from build123d import *

# Parameters (mm, degrees)
SKETCH1_W                      = 40
SKETCH1_H                      = 10.5
BOSS_EXTRUDE1_DEPTH            = 2
SKETCH2_W                      = 14.65
SKETCH2_H                      = 10.5
SKETCH2_W_2                    = 5.2
BOSS_EXTRUDE2_DEPTH            = 3
SKETCH3_W                      = 25
SKETCH3_H                      = 18
BOSS_EXTRUDE3_DEPTH            = 12
CBORE_FOR_M5_SHCS1_D           = 5.5
CBORE_FOR_M5_SHCS1_DEPTH       = 12
CBORE_FOR_M5_SHCS1_CBORE_D     = 10.5
CBORE_FOR_M5_SHCS1_CBORE_DEPTH = 6
FILLET1_R                      = 3
SKETCH6_R                      = 0.95
CUT_EXTRUDE1_DEPTH             = 23


with BuildPart() as part:
    # Sketch1 → Boss-Extrude1 (new body)
    with BuildSketch(Plane.XY):
        with Locations((-20, 5.25)):
            Rectangle(SKETCH1_W, SKETCH1_H)
    extrude(amount=BOSS_EXTRUDE1_DEPTH)

    # Sketch2 → Boss-Extrude2 (add)
    with BuildSketch(Plane.XY.offset(2)):
        with Locations((-32.675, 5.25)):
            Rectangle(SKETCH2_W, SKETCH2_H)
        with Locations((-2.6, 5.25)):
            Rectangle(SKETCH2_W_2, SKETCH2_H)
    extrude(amount=BOSS_EXTRUDE2_DEPTH)

    # Sketch3 → Boss-Extrude3 (add)
    with BuildSketch(Plane(origin=(0, 0, 0), x_dir=(0, 0, -1), z_dir=(1, 0, 0))):
        with Locations((7.5, 9)):
            Rectangle(SKETCH3_W, SKETCH3_H)
    extrude(amount=BOSS_EXTRUDE3_DEPTH)

    # CBORE for M5 SHCS1
    with Locations(Plane(origin=(12, 0, 0), x_dir=(0, 0, -1), z_dir=(1, 0, 0))):
        with Locations((10, 6)):
            CounterBoreHole(CBORE_FOR_M5_SHCS1_D / 2, CBORE_FOR_M5_SHCS1_CBORE_D / 2, CBORE_FOR_M5_SHCS1_CBORE_DEPTH, depth=CBORE_FOR_M5_SHCS1_DEPTH)

    # Fillet1
    fillet1_edges = [part.edges().sort_by_distance(p)[0] for p in [
        (-40, 5.25, 5),
        (12, 9, 5),
        (12, 9, -20),
    ]]
    fillet(fillet1_edges, radius=FILLET1_R)

    # Sketch6 → Cut-Extrude1 (cut, through all)
    with BuildSketch(Plane.XY.offset(2)):
        with Locations((-20.15, 8.022701753)):
            Circle(SKETCH6_R)
        with Locations((-10.65, 8.022701753)):
            Circle(SKETCH6_R)
    extrude(amount=-CUT_EXTRUDE1_DEPTH, mode=Mode.SUBTRACT)


solid = part.part
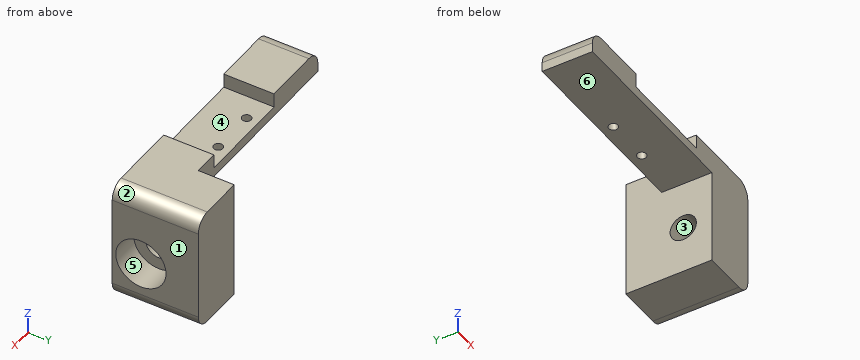
Geometry: final body of the model. Coordinates: model frame, mm. Face numbers are marked on the shaded views. A direction names the side the tool comes from. Coordinates: 2 decimals unless noted, no trailing zeros. Loops run counter-clockwise (first coordinate to the right, second up) from the corner with the lowest first, then second, coordinate; pieces in that order, holes last. Notation, with made-up numbers: (87, -0.75) - (91, -0.75) arc R11 ccw to (91, 10.25) - close; hole circle Ø7 at (44.5, -39). An arc over 180 degrees is marked (long way). One line per question, with ' | ' between items. Start each with the question number.
(1) Cut plane A-A on y = 6. Output: boundary loops of the cut face in (x, z), and give its area (3 significant figures).
(2) Cut plane D-D on z = 0.75. Output: boundary loops of the cut face in (x, y).
(3) Cut plane C-C on x = -10.65. Output: boundary loops of the cut face in (y, z), and give its area (3 significant figures).
(4) First-contact query: pin 1 (8 mm diameter, centred on x = -20.5, y = 13.5, fed in from +Z); pin 2 (5.5 mm diameter, centred on y = 9.5, z = -4, fed in from -X); pin 3 (1.5 mm diameter, centred on x = -17, z = 3.5, fed in from +Y); pin 4 (1.5 mm diameter, centred on y = 6, z = 3, fed in from +X). Flat tips, straight axial feed; report the tip coordinate or a pass-through.
(5) Ray query, L1, parallel to Y at x = 10.1, z = -10; L2, parallel to Y at x = 3.65, z = -10; L3, parallel to X at y = 12, z = -10.5. Return the intervals inside material, ascending. Write a range as from..to.
(6) Cut plane B-B on z = -10. Output: boundary loops of the cut face in (x, y), and give its area (3 significant figures).
(7) Draft query along Z for the marked faces 1, 2 and 3. Return one class per face: +Z half, -Z half, draft (parallel to the pull), parting line (faces both ways), or undercut.
(8) Reachability of the marked faces 4, 5 and 6 from +Z, -Z, +X, -X, +Y, -Y: full face, straight path, thin tool, end or side. Return the list, or none.
Here are the results:
1) outline: (-40, 0) - (0, 0) - (0, -7.25) - (6, -7.25) - (6, -4.75) - (12, -4.75) - (12, 2) arc R3 ccw to (9, 5) - (-5.2, 5) - (-5.2, 2) - (-25.35, 2) - (-25.35, 5) - (-37, 5) arc R3 ccw to (-40, 2) - close; (0, -20) - (9, -20) arc R3 ccw to (12, -17) - (12, -15.25) - (6, -15.25) - (6, -12.75) - (0, -12.75) - close | area: 338 mm²
2) outline: (-40, 0) - (12, 0) - (12, 18) - (0, 18) - (0, 10.5) - (-40, 10.5) - close; hole circle Ø1.9 at (-20.15, 8.02); hole circle Ø1.9 at (-10.65, 8.02)
3) outline: (0, 0) - (7.07, 0) - (7.07, 2) - (0, 2) - close; (8.97, 0) - (10.5, 0) - (10.5, 2) - (8.97, 2) - close | area: 17.2 mm²
4) pin 1: z = 2 | pin 2: x = 0 | pin 3: through | pin 4: x = 11.99
5) L1: 0..0.75, 11.25..18 | L2: 0..3.25, 8.75..18 | L3: 0..12
6) outline: (0, 0) - (12, 0) - (12, 0.75) - (6, 0.75) - (6, 3.25) - (0, 3.25) - close; (0, 8.75) - (6, 8.75) - (6, 11.25) - (12, 11.25) - (12, 18) - (0, 18) - close | area: 120 mm²
7) face 1: draft | face 2: +Z half | face 3: undercut
8) face 4: +Z, +Y, -Y | face 5: +X | face 6: -Z, -X, +Y, -Y
